```python
from build123d import *

# Parameters (mm, degrees)
SKETCH1_W           = 75.7
SKETCH1_H           = 42.7
SKETCH1_R           = 1.75
BOSS_EXTRUDE1_DEPTH = 4
SKETCH3_W           = 75.7
SKETCH3_H           = 29.75
SKETCH3_R           = 1.75
BOSS_EXTRUDE2_DEPTH = 4
SKETCH3_3_R         = 1.75
CUT_EXTRUDE1_DEPTH  = 4
SKETCH4_W           = 75.7
SKETCH4_H           = 40
SKETCH4_R           = 1.75
BOSS_EXTRUDE3_DEPTH = 4
BOSS_EXTRUDE4_DEPTH = 4
SKETCH6_3_R         = 1.75
CUT_EXTRUDE2_DEPTH  = 103.587572347
SKETCH7_W           = 9.15
SKETCH7_H           = 10
SKETCH7_R           = 1.75
BOSS_EXTRUDE5_DEPTH = 4


with BuildPart() as part:
    # Sketch1 → Boss-Extrude1 (new body)
    with BuildSketch(Plane(origin=(0, 0, 0), x_dir=(1, 0, 0), z_dir=(0, 1, 0))):
        Rectangle(SKETCH1_W, SKETCH1_H)
        with Locations(Location((2.4, 17.25, 0), (0, 0, 270))):
            Circle(SKETCH1_R, mode=Mode.SUBTRACT)
        with Locations(Location((-33.8, -17.05, 0), (0, 0, 270))):
            Circle(SKETCH1_R, mode=Mode.SUBTRACT)
        with Locations(Location((29.5, -17.05, 0), (0, 0, 270))):
            Circle(SKETCH1_R, mode=Mode.SUBTRACT)
        with Locations(Location((33.9, 17.25, 0), (0, 0, 270))):
            Circle(SKETCH1_R, mode=Mode.SUBTRACT)
    extrude(amount=BOSS_EXTRUDE1_DEPTH)

    # Sketch3 → Boss-Extrude2 (add)
    with BuildSketch(Plane(origin=(0, 4, 0), x_dir=(1, 0, 0), z_dir=(0, 1, 0))):
        with Locations((0, -36.225)):
            Rectangle(SKETCH3_W, SKETCH3_H)
        with Locations(Location((0, -42.2, 0), (0, 0, 270))):
            Circle(SKETCH3_R, mode=Mode.SUBTRACT)
        with Locations(Location((0, -27.2, 0), (0, 0, 270))):
            Circle(SKETCH3_R, mode=Mode.SUBTRACT)
    extrude(amount=-BOSS_EXTRUDE2_DEPTH)

    # Sketch3_3 → Cut-Extrude1 (cut)
    with BuildSketch(Plane(origin=(0, 4, 0), x_dir=(1, 0, 0), z_dir=(0, 1, 0))):
        with Locations(Location((0, 5.6, 0), (0, 0, 270))):
            Circle(SKETCH3_3_R)
        with Locations(Location((0, -9.4, 0), (0, 0, 270))):
            Circle(SKETCH3_3_R)
    extrude(amount=-CUT_EXTRUDE1_DEPTH, mode=Mode.SUBTRACT)

    # Sketch4 → Boss-Extrude3 (add)
    # profile 1 of 2: a face of its own
    with BuildSketch(Plane(origin=(0, 0, 0), x_dir=(1, 0, 0), z_dir=(0, 1, 0))):
        with Locations((0, -71.1)):
            Rectangle(SKETCH4_W, SKETCH4_H)
        with Locations(Location((-32.85, -53.6, 0), (0, 0, 270))):
            Circle(SKETCH4_R, mode=Mode.SUBTRACT)
        with Locations(Location((-17.85, -53.6, 0), (0, 0, 270))):
            Circle(SKETCH4_R, mode=Mode.SUBTRACT)
        with Locations(Location((-17.85, -88.6, 0), (0, 0, 270))):
            Circle(SKETCH4_R, mode=Mode.SUBTRACT)
        with Locations(Location((-32.85, -88.6, 0), (0, 0, 270))):
            Circle(SKETCH4_R, mode=Mode.SUBTRACT)
        with Locations(Location((32.85, -88.6, 0), (0, 0, 90))):
            Circle(SKETCH4_R, mode=Mode.SUBTRACT)
        with Locations(Location((17.85, -88.6, 0), (0, 0, 90))):
            Circle(SKETCH4_R, mode=Mode.SUBTRACT)
        with Locations(Location((17.85, -53.6, 0), (0, 0, 90))):
            Circle(SKETCH4_R, mode=Mode.SUBTRACT)
        with Locations(Location((32.85, -53.6, 0), (0, 0, 90))):
            Circle(SKETCH4_R, mode=Mode.SUBTRACT)
    # profile 2 of 2: a face of its own
    with BuildSketch(Plane(origin=(0, 0, 0), x_dir=(1, 0, 0), z_dir=(0, 1, 0))):
        Polygon((-37.85, 21.35), (-44, 21.35), (-44, 29.35), (44, 29.35), (44, 21.35), (37.85, 21.35), align=None)
    extrude(amount=BOSS_EXTRUDE3_DEPTH)

    # Sketch6 → Boss-Extrude4 (add)
    with BuildSketch(Plane(origin=(0, 4, 0), x_dir=(1, 0, 0), z_dir=(0, 1, 0))):
        with BuildLine():
            Line((-44, 27.1), (-44, 29.35))
            Line((-44, 29.35), (-47, 29.35))
            Line((-47, 29.35), (-47, 21.35))
            Line((-47, 21.35), (-44, 21.35))
            Line((-44, 21.35), (-44, 23.6))
            ThreePointArc((-44, 23.6), (-45.75, 25.35), (-44, 27.1))
        make_face()
        with BuildLine():
            Line((47, 29.35), (44, 29.35))
            Line((44, 29.35), (44, 27.1))
            ThreePointArc((44, 27.1), (45.75, 25.35), (44, 23.6))
            Line((44, 23.6), (44, 21.35))
            Line((44, 21.35), (47, 21.35))
            Line((47, 21.35), (47, 29.35))
        make_face()
    extrude(amount=-BOSS_EXTRUDE4_DEPTH)

    # Sketch6_3 → Cut-Extrude2 (cut, through all)
    with BuildSketch(Plane(origin=(0, 4, 0), x_dir=(1, 0, 0), z_dir=(0, 1, 0))):
        with Locations(Location((0, 25.35, 0), (0, 0, 270))):
            Circle(SKETCH6_3_R)
        with Locations(Location((22, 25.35, 0), (0, 0, 270))):
            Circle(SKETCH6_3_R)
        with Locations(Location((44, 25.35, 0), (0, 0, 270))):
            Circle(SKETCH6_3_R)
        with Locations(Location((-22, 25.35, 0), (0, 0, 270))):
            Circle(SKETCH6_3_R)
        with Locations(Location((-44, 25.35, 0), (0, 0, 270))):
            Circle(SKETCH6_3_R)
    extrude(amount=-CUT_EXTRUDE2_DEPTH, mode=Mode.SUBTRACT)

    # Sketch7 → Boss-Extrude5 (add)
    # profile 1 of 2: a face of its own
    with BuildSketch(Plane(origin=(0, 0, 0), x_dir=(1, 0, 0), z_dir=(0, 1, 0))):
        with Locations((-42.425, 16.35)):
            Rectangle(SKETCH7_W, SKETCH7_H)
        with Locations(Location((-42.5, 16.35, 0), (0, 0, 270))):
            Circle(SKETCH7_R, mode=Mode.SUBTRACT)
    # profile 2 of 2: a face of its own
    with BuildSketch(Plane(origin=(0, 0, 0), x_dir=(1, 0, 0), z_dir=(0, 1, 0))):
        with Locations((42.425, 16.35)):
            Rectangle(SKETCH7_W, SKETCH7_H)
        with Locations(Location((42.5, 16.35, 0), (0, 0, 270))):
            Circle(SKETCH7_R, mode=Mode.SUBTRACT)
    extrude(amount=BOSS_EXTRUDE5_DEPTH)


solid = part.part
```
Build history of the part. All positions in model axes, mm. A direction names the side the tool comes from. Round coordinates to 2 decimals unless told otherwise and drop trailing zeros. Loops run counter-clockwise (first coordinate to the right, second up) from the corner with the lowest first, then second, coordinate; pieces in that order, holes last.
Item 1: Which spindle directions (+Z, -Z, +X, -X, +Y, -Y) get a long thin tool onto all of the face, cutting with end or side? Do faces 1 (the face through (42, 2, -11.35)), 2 (the face through (33.98, 1.97, -19)). Say none if no direction does.
Item 2: Drill centre lines: line 1 along X through (y, z) = (1.7, -25.35); line 2 along X through (y, z) = (2.05, 88.6); line 3 along Z through (x, y) = (17.85, 3.1). Where is each one in solid material? Low to high.
Item 3: Saw through at C-C (z = 9.4). List the corners of the cut face in (x, y).
Item 4: Saw through at A-A (z = 53.6). List the corners of the cut face in (x, y).
Item 5: Pin check, flat tips, straight feed: P1, Ø3, axis at x = 0, z = -5.6, coming from the +Y side; P2, Ø2, axis at y = 3, z = 22.5, coming from the +X side. Stop position of each tip, or through.
Item 6: Two-plate mould, pull along X, no slides. Class faces 3 (the face through (-1.06, 2.03, 25.81)), 4 (the face through (37.85, 2, 41)), 5 (the face through (-1, 0, 30)), 6 (the face through (-47, 2, -20)): released by +X, released by -X, zero draft, split by the parting line, or undercut.
Item 7: Saw through at B-B (x = 17.85). List the corners of the cut face in (y, z), then the cut area to 3 significant figures.
Item 8: Saw through at D-D (x = 29.5). List the corners of the cut face in (y, z).
Worked answers:
1. face 1: +Z, +X, +Y, -Y
1. face 2: +Y, -Y
2. line 1: x = -47 to -45.75, -42.25 to -23.75, -20.25 to -1.75, 1.75 to 20.25, 23.75 to 42.25, 45.75 to 47
2. line 2: x = -37.85 to -34.6, -31.1 to -19.6, -16.1 to 16.1, 19.6 to 31.1, 34.6 to 37.85
2. line 3: z = -29.35 to 51.85, 55.35 to 86.85, 90.35 to 91.1
3. outline: (-37.85, 0) - (-1.75, 0) - (-1.75, 4) - (-37.85, 4) - close; (1.75, 0) - (37.85, 0) - (37.85, 4) - (1.75, 4) - close
4. outline: (-37.85, 0) - (-34.6, 0) - (-34.6, 4) - (-37.85, 4) - close; (-31.1, 0) - (-19.6, 0) - (-19.6, 4) - (-31.1, 4) - close; (-16.1, 0) - (16.1, 0) - (16.1, 4) - (-16.1, 4) - close; (19.6, 0) - (31.1, 0) - (31.1, 4) - (19.6, 4) - close; (34.6, 0) - (37.85, 0) - (37.85, 4) - (34.6, 4) - close
5. P1: passes through
5. P2: stops at x = 37.85
6. face 3: undercut
6. face 4: released by +X
6. face 5: zero draft
6. face 6: released by -X
7. outline: (0, -29.35) - (4, -29.35) - (4, 51.85) - (0, 51.85) - close; (0, 55.35) - (4, 55.35) - (4, 86.85) - (0, 86.85) - close; (0, 90.35) - (4, 90.35) - (4, 91.1) - (0, 91.1) - close
7. area: 454 mm2
8. outline: (0, -29.35) - (4, -29.35) - (4, 15.3) - (0, 15.3) - close; (0, 18.8) - (4, 18.8) - (4, 91.1) - (0, 91.1) - close
